Design review of the part shown in the three views and the two pictorial views. Dimensions are in mm from the part's minimum x, y and z. Coordinates: 2 decimals unless noted, no trailing zeros. Write each loop counter-clockwise with the first axis right and the second up, starting at its lowest first coordinate (ties: lowest second). Pieces come first, ordered by that corner, then holes. Notation, with made-up numbers: (45.25, 37) -> (73.25, 37) arc R20 ccw to (73.25, 76) -> close; hole circle Ø1 at (1, -16.5). An arc over 180 degrees is marked (long way). Write each question's results on one line, items separated by ' | '.
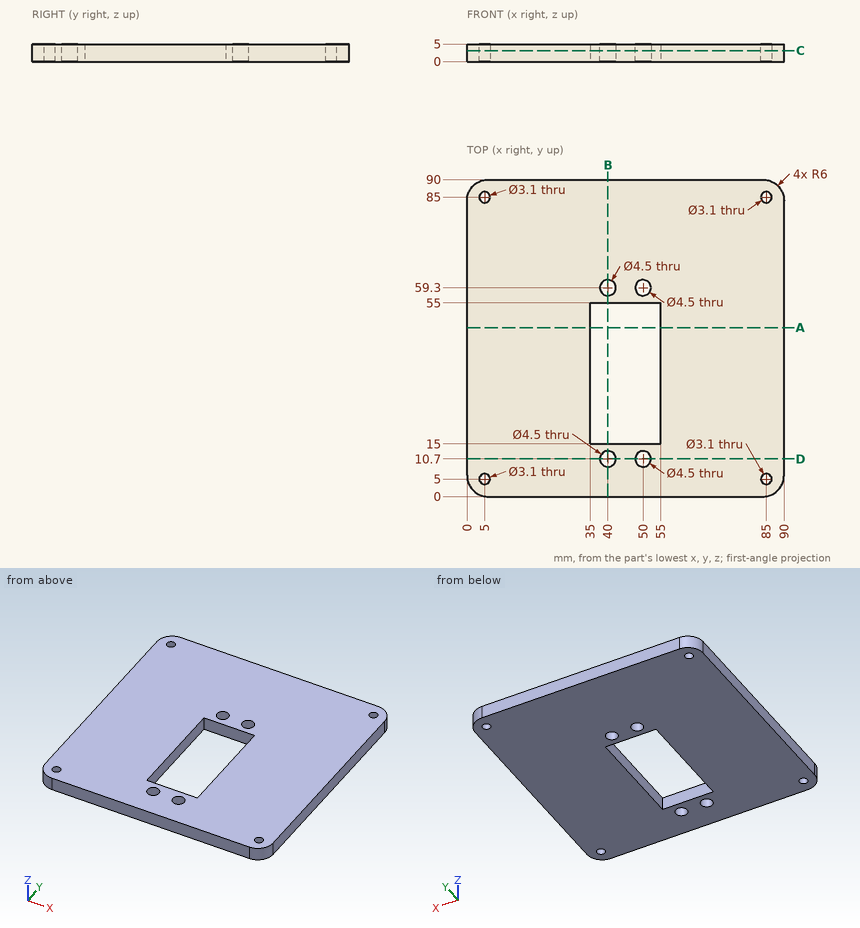
Q1. Add section A-A (y = 48). Write out the cut boundary in (x, z).
Solution:
outline: (0, 0) -> (35, 0) -> (35, 5) -> (0, 5) -> close; (55, 0) -> (90, 0) -> (90, 5) -> (55, 5) -> close
Q2. Add section D-D (y = 10.7). Write out the cut boundary in (x, z), plus the area to 3 significant figures.
Solution:
outline: (0, 0) -> (37.75, 0) -> (37.75, 5) -> (0, 5) -> close; (42.25, 0) -> (47.75, 0) -> (47.75, 5) -> (42.25, 5) -> close; (52.25, 0) -> (90, 0) -> (90, 5) -> (52.25, 5) -> close | area: 405 mm²
Q3. Add section B-B (x = 40). Write out the cut boundary in (y, z), plus the area to 3 significant figures.
Solution:
outline: (0, 0) -> (8.45, 0) -> (8.45, 5) -> (0, 5) -> close; (12.95, 0) -> (15, 0) -> (15, 5) -> (12.95, 5) -> close; (55, 0) -> (57.05, 0) -> (57.05, 5) -> (55, 5) -> close; (61.55, 0) -> (90, 0) -> (90, 5) -> (61.55, 5) -> close | area: 205 mm²
Q4. For line 1 (Y direction, x = 40, z = 3.65); line 2 (X direction, y = 41.5, z = 3.2); line 3 (X direction, y = 11, z = 2.85), list the stretches that pass through material, from the lowest coordinate up. Write a range as from..to.
Solution:
line 1: 0..8.45, 12.95..15, 55..57.05, 61.55..90 | line 2: 0..35, 55..90 | line 3: 0..37.77, 42.23..47.77, 52.23..90
Q5. Add section C-C (z = 3.1). Count the separate pieces of the cut face and the enclosed holes in it, plus the area to 3 significant figures.
Solution:
separate pieces: 1 | enclosed holes: 9 | area: 7,180 mm²
